Could you check a few things on this model? Use its own coordinates, in mm. A direction names the side the tool comes from. Round coordinates to 2 decimals unless told otherwise and drop trailing zeros. Write each loop counter-clockwise with the first axis right and the second up, starting at its lowest first coordinate (ties: lowest second). Pieces come first, ordered by that corner, then holes. Notation, with made-up numbers: (-33, 61.25) -> (-27, 61.25) arc R21 cw to (-27, 79.25) -> close; hole circle Ø3 at (51.5, 83.25). An arc over 180 degrees is marked (long way). Answer in a Markdown table with one row per item.
from build123d import *

# Parameters (mm, degrees)
SKETCH_2_W          = 15.2
SKETCH_2_H          = 15.2
CUT_EXTRUDE_1_DEPTH = 25


with BuildPart() as part:
    # Эскиз1 → Повернуть1 (revolve)
    with BuildSketch(Plane.XY, mode=Mode.PRIVATE) as revolve_1_sk:
        Polygon((0, 20), (3, 20), (3, 35), (4.15, 35), (4.15, 31.5), (5.65, 31.5), (5.65, 30.5), (12.65, 30.5), (12.65, 0), (0, 0), align=None)
    revolve(revolve_1_sk.sketch.rotate(Axis((0, 0, 0), (0, 1, 0)), 90), axis=Axis((0, 0, 0), (0, 1, 0)))

    # Эскиз2 → Вырез-Вытянуть1 (cut)
    with BuildSketch(Plane.XZ):
        Rectangle(SKETCH_2_W, SKETCH_2_H)
    extrude(amount=-CUT_EXTRUDE_1_DEPTH, mode=Mode.SUBTRACT)


solid = part.part
1) For pin 1 (1 mm diameter, centred on x = 3, y = 10.5, fed in from -Z); pin 2 (4 mm diameter, centred on x = 8.5, z = 6, fed in from +Y); pin 3 (1 mm diameter, centred on x = 1, y = 28, fed in from -Z), each with a flat end and sliding along its axis, tell me the tip position at first contact or that it passes through.
Findings:
| item | result |
|---|---|
| pin 1 | stops at z = -12.4 |
| pin 2 | stops at y = 30.5 |
| pin 3 | stops at z = -12.64 |
2) Imagine slicing it at A-A, the plane z = 0. Please give me the cut outline in (x, y), plus the area to 3 significant figures.
Findings:
| item | result |
|---|---|
| outline | (-12.65, 0) -> (-7.6, 0) -> (-7.6, 25) -> (-3, 25) -> (-3, 35) -> (-4.15, 35) -> (-4.15, 31.5) -> (-5.65, 31.5) -> (-5.65, 30.5) -> (-12.65, 30.5) -> close; (3, 25) -> (7.6, 25) -> (7.6, 0) -> (12.65, 0) -> (12.65, 30.5) -> (5.65, 30.5) -> (5.65, 31.5) -> (4.15, 31.5) -> (4.15, 35) -> (3, 35) -> close |
| area | 372 mm^2 |
3) Thinking about a two-plate mould opening in Z: for faces 1 (the face through (3, 30.5, 5)), 2 (the face through (0, 12, 7.6)), 3 (the face through (-1.7, 30.99, -5.39)), which applies, +Z half, -Z half, draft (parallel to the pull), parting line (faces both ways), or undercut?
Findings:
| item | result |
|---|---|
| face 1 | draft |
| face 2 | undercut |
| face 3 | parting line |
4) Please list where these lines run through material, in increasing order: line 1 (X direction, y = 33.25, z = 0); line 2 (Y direction, x = -7.25, z = -7.5); line 3 (X direction, y = 10.5, z = 7.5).
Findings:
| item | result |
|---|---|
| line 1 | x = -4.15 to -3, 3 to 4.15 |
| line 2 | y = 25 to 30.5 |
| line 3 | x = -10.19 to -7.6, 7.6 to 10.19 |
5) Imagine slicing it at D-D, the plane z = -10.5. Please give me the cut outline in (x, y), plus the area to 3 significant figures.
Findings:
| item | result |
|---|---|
| outline | (-7.05, 0) -> (7.05, 0) -> (7.05, 30.5) -> (-7.05, 30.5) -> close |
| area | 430 mm^2 |
6) Imagine slicing it at B-B, the plane x = 0. Please give me the cut outline in (y, z).
Findings:
| item | result |
|---|---|
| outline | (0, -12.65) -> (30.5, -12.65) -> (30.5, -5.65) -> (31.5, -5.65) -> (31.5, -4.15) -> (35, -4.15) -> (35, -3) -> (25, -3) -> (25, -7.6) -> (0, -7.6) -> close; (0, 7.6) -> (25, 7.6) -> (25, 3) -> (35, 3) -> (35, 4.15) -> (31.5, 4.15) -> (31.5, 5.65) -> (30.5, 5.65) -> (30.5, 12.65) -> (0, 12.65) -> close |
7) For faces 4 (the face through (-7.6, 12, 0)), 5 (the face through (4.05, 33.23, 0.9)), 6 (the face through (12.35, 15.04, 2.74)), which set-ups out of +Z, -Z, +X, -X, +Y, -Y let a thin tool reach every point of the face, with its end or its side?
Findings:
| item | result |
|---|---|
| face 4 | -Y |
| face 5 | +Y |
| face 6 | +Y, -Y |
8) Imagine slicing it at C-C, the plane y = 12.5. Please give me the cut outline in (x, z).
Findings:
| item | result |
|---|---|
| outline | circle Ø25.3 at (0, 0); hole (-7.6, -7.6) -> (7.6, -7.6) -> (7.6, 7.6) -> (-7.6, 7.6) -> close |
